Check sheet for the drawn part. Datum: minimum x, y, z corner. Units: mm. A direction names the side the tool comes from. Round coordinates to 2 decimals unless told otherwise and drop trailing zeros. Write each loop counter-clockwise with the first axis right and the second up, starting at its lowest first coordinate (ties: lowest second). Pieces come first, ordered by that corner, then holes.
Item 1: Cross-section at B-B on z = 15. Enter the section's corners in (x, y), plus the area to 3 significant figures.
Item 2: Cross-section at A-A on y = 36. Enter the section's corners in (x, z), plus the area to 3 significant figures.
Item 3: Cross-section at D-D on y = 19. Enter the section's corners in (x, z).
Item 4: Material ranges on line 1 (Z direction, x = 30, y = 3); line 2 (X direction, y = 36.5, z = 2); line 3 (X direction, y = 30, z = 25.25), recorded low to high.
Item 5: Tool access check on the marked faces 1, 2 and 3. Record the directions out of +Z, -Z, +X, -X, +Y, -Y that give a thin tool (end or side, any length) a straight path to the whole face; none if there is none.
Item 6: Go/stop test with flat-tipped pins: pin 1 Ø8.5 at (y, z) = (39.5, 26) entering from -X; pin 2 Ø6 at (x, y) = (50, 28) entering from -Z; pin 3 Ø3.5 at (x, z) = (52.5, 17) entering from +Y; pin 4 Ø6 at (x, z) = (8, 7) entering from +Y. Record where each tip stops, or that it passes through.
Item 7: Cross-section at C-C on x = 12. Enter the section's corners in (y, z), plus the area to 3 significant figures.
Item 8: Release check for a two-part mould opening along X. For the marked faces 4, 5, 6 and 7 record: +X half, -X half, draft (parallel to the pull), parting line (faces both ways), or undercut.
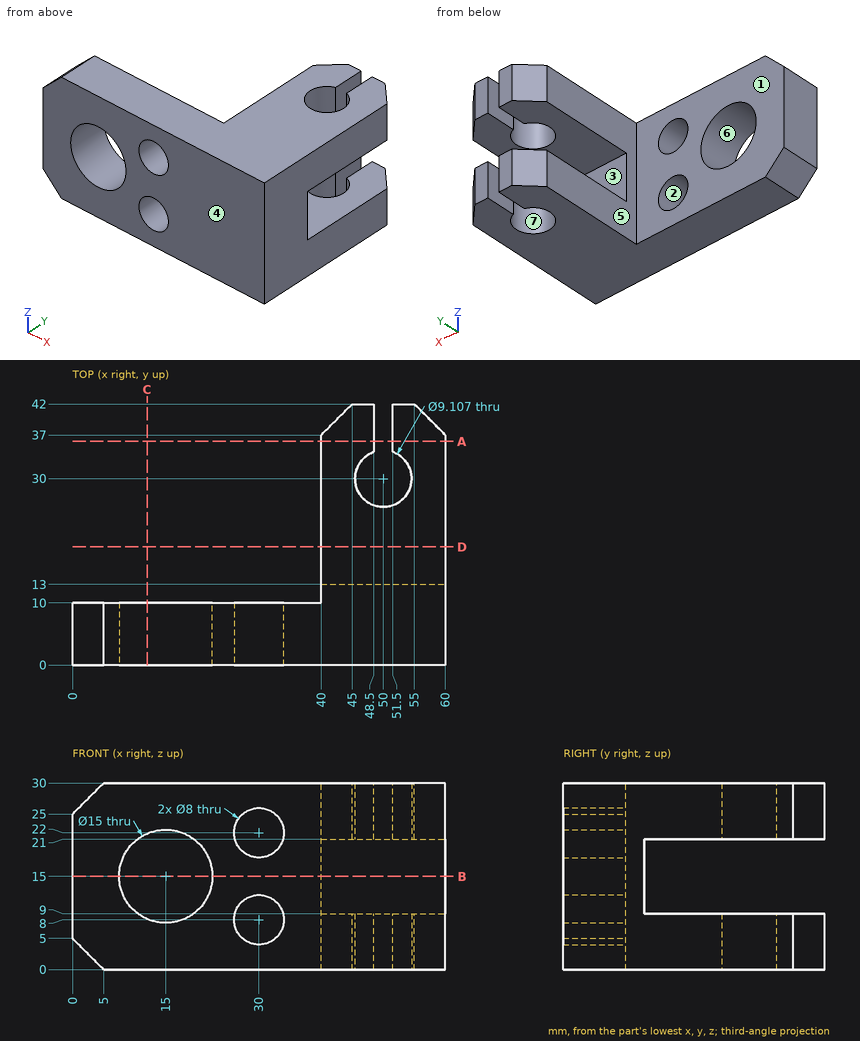
Response values:
1. outline: (0, 0) - (7.5, 0) - (7.5, 10) - (0, 10) - close; (22.5, 0) - (60, 0) - (60, 13) - (40, 13) - (40, 10) - (22.5, 10) - close
1. area: 510 mm2
2. outline: (40, 0) - (48.5, 0) - (48.5, 9) - (40, 9) - close; (40, 21) - (48.5, 21) - (48.5, 30) - (40, 30) - close; (51.5, 0) - (60, 0) - (60, 9) - (51.5, 9) - close; (51.5, 21) - (60, 21) - (60, 30) - (51.5, 30) - close
2. area: 306 mm2
3. outline: (40, 0) - (60, 0) - (60, 9) - (40, 9) - close; (40, 21) - (60, 21) - (60, 30) - (40, 30) - close
4. line 1: z = 0 to 4, 12 to 18, 26 to 30
4. line 2: x = 40 to 48.5, 51.5 to 60
4. line 3: x = 40 to 45.45, 54.55 to 60
5. face 1: +Z, -Z, -X, +Y
5. face 2: +Y, -Y
5. face 3: +X, -X, +Y
6. pin 1: stops at x = 40
6. pin 2: stops at z = 0
6. pin 3: stops at y = 13
6. pin 4: stops at y = 10
7. outline: (0, 0) - (10, 0) - (10, 8.13) - (0, 8.13) - close; (0, 21.87) - (10, 21.87) - (10, 30) - (0, 30) - close
7. area: 163 mm2
8. face 4: draft
8. face 5: -X half
8. face 6: undercut
8. face 7: undercut
